```python
from build123d import *

# Parameters (mm, degrees)
F0_W     = 38.1
F0_H     = 88.9
F1_DEPTH = 1409.7
F2_W     = 88.9
F2_H     = 19.05
F3_DEPTH = 88.9


with BuildPart() as f1:
    # F0 (on Right) → F1 (new body)
    with BuildSketch(Plane.YZ):
        Rectangle(F0_W, F0_H)
    extrude(amount=F1_DEPTH)

    # F2 (on face) → F3 (cut, through all)
    with BuildSketch(Plane.XY.offset(44.45)):
        with Locations((958.85, -9.525)):
            Rectangle(F2_W, F2_H)
    extrude(amount=-F3_DEPTH, mode=Mode.SUBTRACT)

    # F4: F1 across plane


with BuildPart() as f1_1:
    add(f1.part)
    add(f1.part.mirror(Plane.YZ))


solid = f1_1.part
```
Can you work these out from the model? Positions are in its coordinate system, mm. A direction names the side the tool comes from. Coordinates: 2 decimals unless noted, no trailing zeros. Loops run counter-clockwise (first coordinate to the right, second up) from the corner with the lowest first, then second, coordinate; pieces in that order, holes last.
1) I need wall thicknesses on probe 1 along X at (y, z) = (-5, -24); probe 2 along Y at (x, z) = (928.5, 24.5). Which ranges of each line are inside material? Lowest first, please.
2) Which directions (+Z, -Z, +X, -X, +Y, -Y) give clear straight access to the entire face, cutting with the end or side of a thin tool? Please do faces 1 (the flat face through (-958, 0, 1)), 2 (the flat face through (20, 19.05, -1)).
3) Imagine slicing it at A-A on z = -17. List the corners of the cut face in (x, y) for me, plus the area to 3 significant figures.
Completed:
1. probe 1: x = -1409.7 to -1003.3, -914.4 to 914.4, 1003.3 to 1409.7
1. probe 2: y = 0 to 19.05
2. face 1: +Z, -Z, -Y
2. face 2: +Z, -Z, +X, -X, +Y
3. outline: (-1409.7, -19.05) - (-1003.3, -19.05) - (-1003.3, 0) - (-914.4, 0) - (-914.4, -19.05) - (914.4, -19.05) - (914.4, 0) - (1003.3, 0) - (1003.3, -19.05) - (1409.7, -19.05) - (1409.7, 19.05) - (-1409.7, 19.05) - close
3. area: 104,000 mm2
